The model under review builds one solid part; all positions refer to its coordinate system, in mm. Face numbers are marked on the shaded views. Round coordinates to 2 decimals unless told otherwise and drop trailing zeros. Write each loop counter-clockwise with the first axis right and the second up, starting at its lowest first coordinate (ties: lowest second). Pieces come first, ordered by that corner, then holes. Notation, with made-up numbers: M 77.25,48.25 L 82.25,48.25 A7 ccw 82.25,55.25 Z; hole C 45,33 d9. An arc over 180 degrees is marked long. One line per item, written item: value. Start each with the question number.
1) Take a section at A-A, the plane x = 0. Write out the cut boundary in (y, z), and give its area (3 significant figures).
2) Take a section at C-C, the plane z = 1.1. Write out the cut boundary in (x, y), and give its area (3 significant figures).
3) Wall thickness on probe 1 along Z at (x, y) = (0, 9.5); probe 2 along X at (y, z) = (1.5, 0.5); probe 3 along X at (y, z) = (6.75, 1.2): over which ranges is each line inside the solid? List them lowest first.
4) Mouldability with a two-part tool opening along Z and no side actions: class the marked faces 1, 2 and 3 as +Z half, -Z half, draft (parallel to the pull), parting line (faces both ways), or undercut.
5) For P1, Ø3, axis at x = 0, z = 0, coming from the -Y side, flat-tipped, find the tip position at first contact; note if it passes through.
6) Take a section at B-B, the plane y = 8. Write out the cut boundary in (x, z).
7) Take a section at D-D, the plane z = -2.35. Write out the cut boundary in (x, y).
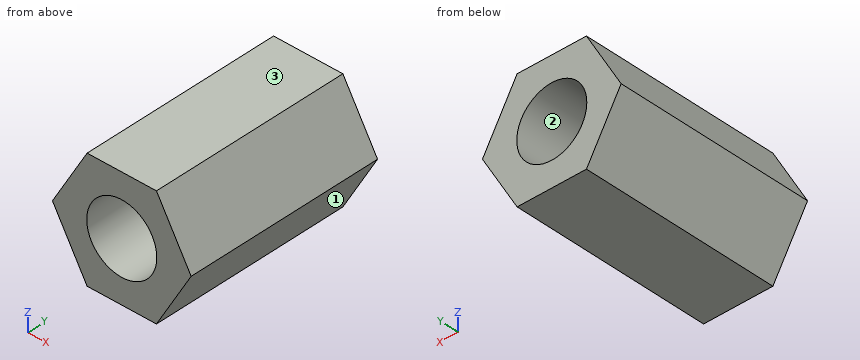
Autodesk Inventor part; units mm, degrees
ref_plane "YZ Plane" through (0, 0, 0) normal (1, 0, 0) x (0, 1, 0)
ref_plane "XZ Plane" through (0, 0, 0) normal (0, 1, 0) x (-1, 0, 0)
ref_plane "XY Plane" through (0, 0, 0) normal (0, 0, 1) x (1, 0, 0)
sketch "Sketch1" plane through (0, 0, 0) normal (0, 1, 0) x (-1, 0, 0)
  circle A0 centre (0, 0) radius 1.75
  line L0 (3.4641, 0) -> (1.7321, -3)
  line L1 (1.7321, -3) -> (-1.7321, -3)
  line L2 (-1.7321, -3) -> (-3.4641, 0)
  line L3 (-3.4641, 0) -> (-1.7321, 3)
  line L4 (-1.7321, 3) -> (1.7321, 3)
  line L5 (1.7321, 3) -> (3.4641, 0)
  point P0 (0, -3)
  point P1 (0, 3)
  dimension "d0" = 3.5
  dimension "d1" = 6
extrude "Extrusion1" add sketch "Sketch1" along normal blind 10
properties part number "Heated Bed Spacer" material "ABS Plastic"
Checked values:
1. outline: M 0,-3 L 10,-3 L 10,-1.75 L 0,-1.75 Z; M 0,1.75 L 10,1.75 L 10,3 L 0,3 Z
1. area: 25.0 mm2
2. outline: M -2.83,0 L -1.36,0 L -1.36,10 L -2.83,10 Z; M 1.36,0 L 2.83,0 L 2.83,10 L 1.36,10 Z
2. area: 29.4 mm2
3. probe 1: z = -3 to -1.75, 1.75 to 3
3. probe 2: x = -3.18 to -1.68, 1.68 to 3.18
3. probe 3: x = -2.77 to -1.27, 1.27 to 2.77
4. face 1: -Z half
4. face 2: undercut
4. face 3: +Z half
5. P1: passes through
6. outline: M -3.46,0 L -1.73,-3 L 1.73,-3 L 3.46,0 L 1.73,3 L -1.73,3 Z; hole C 0,0 d3.5
7. outline: M -2.11,0 L 2.11,0 L 2.11,10 L -2.11,10 Z
